Build history of the part. All positions in model axes, mm. A direction names the side the tool comes from. Give positions to 0.01 mm unless a question says otherwise; leave off trailing zeros. Order: outer loops, then holes, each group sorted by start corner. A loop starts at its lowest first (then second) coordinate and runs counter-clockwise, first axis right, second up. Notation, with made-up numbers: M 1,29.5 L 57,29.5 A25 cw 57,68.5 Z; hole C -9.75,87 d5. An arc over 180 degrees is marked long. Answer as CSV lines item,"result".
from build123d import *

# Parameters (mm, degrees)
SKETCH_1_W          = 70
SKETCH_1_H          = 57.5
EXTRUDE_1_DEPTH     = 22
SKETCH_2_R          = 7.5
EXTRUDE_2_DEPTH     = 15
SKETCH_3_R          = 1
CUT_EXTRUDE_1_DEPTH = 5


with BuildPart() as part:
    # 草图1 → 凸台-拉伸1 (new body)
    with BuildSketch(Plane(origin=(0, 0, 0), x_dir=(1, 0, 0), z_dir=(0, 1, 0))):
        Rectangle(SKETCH_1_W, SKETCH_1_H)
    extrude(amount=EXTRUDE_1_DEPTH)

    # 草图2 → 凸台-拉伸2 (add)
    with BuildSketch(Plane.XY.offset(28.75)):
        with Locations((-22, 11)):
            Circle(SKETCH_2_R)
        with Locations((0, 11)):
            Circle(SKETCH_2_R)
        with Locations((22, 11)):
            Circle(SKETCH_2_R)
    extrude(amount=EXTRUDE_2_DEPTH)

    # 草图3 → 切除-拉伸1 (cut)
    with BuildSketch(Plane.XZ):
        with Locations((-32, 25)):
            Circle(SKETCH_3_R)
        with Locations((-32, -25)):
            Circle(SKETCH_3_R)
        with Locations((32, -25)):
            Circle(SKETCH_3_R)
        with Locations((32, 25)):
            Circle(SKETCH_3_R)
    extrude(amount=-CUT_EXTRUDE_1_DEPTH, mode=Mode.SUBTRACT)


solid = part.part
Item 1: Band-saw the part on D-D (x = -1). Give the cut face in (y, z).
Geometry says:
outline,"M 0,-28.75 L 22,-28.75 L 22,28.75 L 18.43,28.75 L 18.43,43.75 L 3.57,43.75 L 3.57,28.75 L 0,28.75 Z"
Item 2: Band-saw the part on A-A (x = -22). Give the cut face in (y, z).
Geometry says:
outline,"M 0,-28.75 L 22,-28.75 L 22,28.75 L 18.5,28.75 L 18.5,43.75 L 3.5,43.75 L 3.5,28.75 L 0,28.75 Z"
Item 3: Band-saw the part on C-C (z = 35.5). Give the cut face in (x, y), and give its area (3 significant figures).
Geometry says:
outline,"C -22,11 d15; C 0,11 d15; C 22,11 d15"
area,"530 mm2"
Item 4: Probe line 1 along Z through (x, y) = (32, 1.25); line 2 along X through (y, z) = (12, 37); line 3 along Z through (x, y) = (-6.5, 4.75). List the from-to ranges inside material, lowest first. Write a range as from..to.
Geometry says:
line 1,"z = -28.75..-26, -24..24, 26..28.75"
line 2,"x = -29.43..-14.57, -7.43..7.43, 14.57..29.43"
line 3,"z = -28.75..28.75"
Item 5: Band-saw the part on B-B (y = 11). Give the cut face in (x, z), and give its area (3 significant figures).
Geometry says:
outline,"M -35,-28.75 L 35,-28.75 L 35,28.75 L 29.5,28.75 L 29.5,43.75 L 14.5,43.75 L 14.5,28.75 L 7.5,28.75 L 7.5,43.75 L -7.5,43.75 L -7.5,28.75 L -14.5,28.75 L -14.5,43.75 L -29.5,43.75 L -29.5,28.75 L -35,28.75 Z"
area,"4,700 mm2"
Item 6: 3-axis set-ups, long thin cutter, end or side, ignore diameter. For faces 1 (the flat face through (32, 5, 25)), 2 (the cylindrical face through (16.048, 6.436, 36.145)), 3 (the flat face through (22, 11, 43.75)): which of +Z, -Z, +X, -X, +Y, -Y reach the whole face in a straight line?
Geometry says:
face 1,"-Y"
face 2,"+Z"
face 3,"+Z, +X, -X, +Y, -Y"
Item 7: Pull direction X, two halves, no side cores. Call faces 4 (the flat face through (0, 11, -28.75)), 5 (the flat face through (-35, 11, 0)), 6 (the flat face through (-32, 5, -25)): released by +X, released by -X, zero draft, split by the parting line, or undercut.
Geometry says:
face 4,"zero draft"
face 5,"released by -X"
face 6,"undercut"
Item 8: Drop flat-ended pins along their axis: pin 1 (0.6 mm diameter, centred on x = 32, z = 25, fed in from -Y); pin 2 (1 mm diameter, centred on x = 15, z = 30, fed in from -Y); pin 3 (2.5 mm diameter, centred on x = -32, z = -25, fed in from -Y). Give the stop position or say it passes through.
Geometry says:
pin 1,"stops at y = 5"
pin 2,"stops at y = 7.26"
pin 3,"stops at y = 0"
